Verification items for this drawing (mm, ordinates from the low corner). A direction names the side the tool comes from. Give positions to 0.01 mm unless a question says otherwise; leave off trailing zeros. Order: outer loops, then holes, each group sorted by start corner. A loop starts at its lowest first (then second) coordinate and runs counter-clockwise, first axis right, second up.
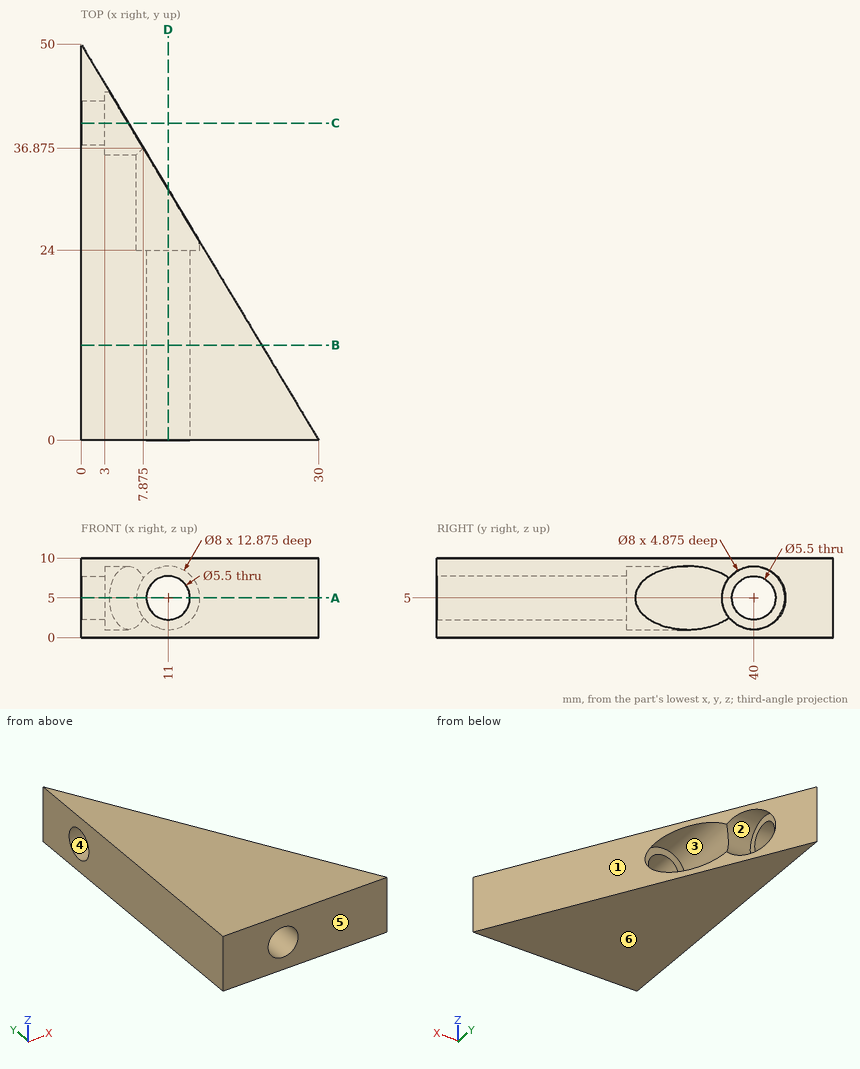
Q1. Cross-section at C-C, the plane y = 40. Record the boundary of the cut face in (x, z), and give its area (3 significant figures).
Q2. Access from +Z, -Z, +X, -X, +Y, -Y to the whole of each face (thin tool, end or side, straight path). Record for the marked faces 1, 2 and 3.
Q3. Thickness scan on L1, parallel to Z at x = 4, y = 40; L2, parallel to X at y = 37.5, z = 2.75; L3, parallel to Z at x = 8.5, y = 12. Record the ranges inside material, lowest first.
Q4. Release check for a two-part mould opening along Y. For the marked faces 4, 5 and 6 record: pulls with the +Y half, pulls with the -Y half, needs draft (parallel to the pull), parting line crosses it, or undercut.
Q5. Cross-section at A-A, the plane z = 5. Record the boundary of the cut face in (x, y), and give its area (3 significant figures).
Q6. Cross-section at B-B, the plane y = 12. Record the boundary of the cut face in (x, z), and give its area (3 significant figures).
Q7. Gauge pin test, flat ends, axial feed: P1, Ø4, axis at x = 23, z = 2.5, coming from the +Y side; P2, Ø2.5, axis at x = 10.5, z = 7, coming from the +Y side; P3, Ø2, axis at y = 34.5, z = 3.5, coming from the +X side. Record the tip position at first contact, or that the pin passes through.
Q8. Cross-section at D-D, the plane x = 11. Record the boundary of the cut face in (y, z), and give its area (3 significant figures).
Answers follow:
1. outline: (0, 0) - (6, 0) - (6, 1) - (3, 1) - (3, 2.25) - (0, 2.25) - close; (0, 7.75) - (3, 7.75) - (3, 9) - (6, 9) - (6, 10) - (0, 10) - close
1. area: 19.5 mm2
2. face 1: +Z, -Z, +X, +Y
2. face 2: +X
2. face 3: +Y
3. L1: z = 0 to 1, 9 to 10
3. L2: x = 0 to 3
3. L3: z = 0 to 3.85, 6.15 to 10
4. face 4: undercut
4. face 5: pulls with the -Y half
4. face 6: needs draft
5. outline: (0, 0) - (8.25, 0) - (8.25, 24) - (7, 24) - (7, 36) - (3, 36) - (3, 37.25) - (0, 37.25) - close; (0, 42.75) - (3, 42.75) - (3, 44) - (3.6, 44) - (0, 50) - close; (13.75, 0) - (30, 0) - (15, 25) - (15, 24) - (13.75, 24) - close
5. area: 518 mm2
6. outline: (0, 0) - (22.8, 0) - (22.8, 10) - (0, 10) - close; hole circle Ø5.5 at (11, 5)
6. area: 204 mm2
7. P1: stops at y = 15
7. P2: stops at y = 24
7. P3: stops at x = 7.88
8. outline: (0, 0) - (31.67, 0) - (31.67, 1) - (24, 1) - (24, 2.25) - (0, 2.25) - close; (0, 7.75) - (24, 7.75) - (24, 9) - (31.67, 9) - (31.67, 10) - (0, 10) - close
8. area: 123 mm2
